For this review, take the finished solid that the model builds, in its own axes (mm). Face numbers are marked on the shaded views. A direction names the side the tool comes from. Coordinates: 2 decimals unless noted, no trailing zeros. Loops run counter-clockwise (first coordinate to the right, second up) from the corner with the lowest first, then second, coordinate; pieces in that order, holes last. Notation, with made-up numbers: (-28.5, 59) - (20.5, 59) arc R18 cw to (20.5, 84) - close; hole circle Ø7 at (46.5, 79.25). An arc over 180 degrees is marked (long way). Answer as a JSON object with one key per item and string values. Group by question number.
Item 1: Tool access review of the marked faces 5, 6 and 7: name each direction out of +Z, -Z, +X, -X, +Y, -Y from which nothing blocks a thin tool from reaching the whole face with its end or side.
Item 2: Clearance check with flat-ended pins moving along their axes: pin 1 (8 mm diameter, centred on x = 8, z = -6.5, fed in from -Y); pin 2 (1 mm diameter, centred on x = -1, z = -1, fed in from -Y); pin 3 (4 mm diameter, centred on x = -7.5, z = 3.5, fed in from -Y); pin 4 (10 mm diameter, centred on x = -3.5, y = -1.5, fed in from -Z). State where each tip first meets the part, or that it passes through.
Item 3: Mouldability with a two-part tool opening along Z and no side actions: class the marked faces 1, 2, 3 and 4 as released by +Z, released by -Z, zero draft, split by the parting line, or undercut.
Item 4: We need section C-C (z = 4.5). Give the boundary of the cut face in (x, y), then the cut area to 3 significant figures.
Item 5: To check wall thickness, follow line 1 (Y direction, x = 0, z = -3.5); line 2 (X direction, y = 3.5, z = 0.5); line 3 (Z direction, x = 6.5, y = 6). State the ranges of each line that lie inside material, in increasing order.
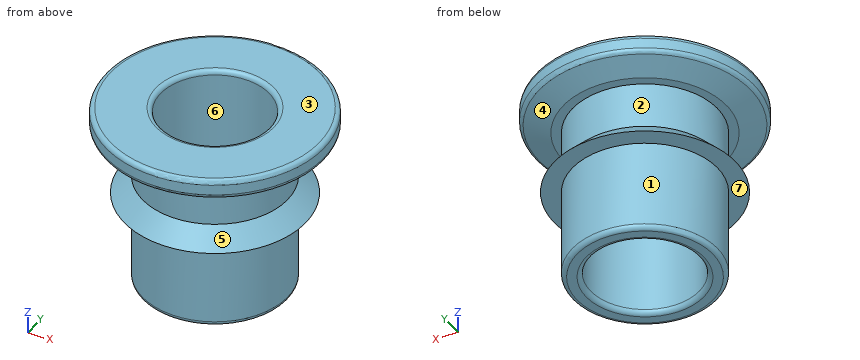
from build123d import *

# Parameters (mm, degrees)
F0_R     = 8
F0_R_2   = 6
F1_DEPTH = 10
F2_R     = 10
F2_R_2   = 6
F3_DEPTH = 2
F4_R     = 8
F4_R_2   = 6
F5_DEPTH = 5
F6_R     = 12
F6_R_2   = 6
F7_DEPTH = 3
F8_SIZE  = 1.99999
F9_SIZE2 = 3
F9_SIZE  = 1


# Not quite as in the source:
# - a fillet or chamfer that OpenCascade refuses, or shapes differently, is made with other operations: its cross-section is extruded or revolved along the edge and cut away or added
# - a fillet or chamfer is up to 0.001 mm smaller than in the source, because OpenCascade refuses the exact size


with BuildPart() as f1:
    # F0 (on Top) → F1 (new body)
    with BuildSketch(Plane.XY):
        Circle(F0_R)
        Circle(F0_R_2, mode=Mode.SUBTRACT)
    extrude(amount=-F1_DEPTH)

    # F2 (on Top) → F3 (join)
    with BuildSketch(Plane.XY):
        Circle(F2_R)
        Circle(F2_R_2, mode=Mode.SUBTRACT)
    extrude(amount=F3_DEPTH)

    # F4 (on face) → F5 (join)
    with BuildSketch(Plane.XY.offset(2)):
        Circle(F4_R)
        Circle(F4_R_2, mode=Mode.SUBTRACT)
    extrude(amount=F5_DEPTH)

    # F6 (on face) → F7 (join)
    with BuildSketch(Plane.XY.offset(7)):
        Circle(F6_R)
        Circle(F6_R_2, mode=Mode.SUBTRACT)
    extrude(amount=F7_DEPTH)

    # F8 (size 2 in the source; OpenCascade refuses exactly that, so slightly less here)
    f8_edges = [f1.edges().sort_by_distance(p)[0] for p in [
        (-10, 0, 2),
    ]]
    chamfer(f8_edges, length=F8_SIZE)

    # F9
    f9_edges = [f1.edges().sort_by_distance(p)[0] for p in [
        (-12, 0, 7),
    ]]
    f9_side = f1.faces().sort_by_distance((-12, 0, 8.5))[0]
    chamfer(f9_edges, length=F9_SIZE, length2=F9_SIZE2, reference=f9_side)

    # F10: fillet of radius 0.5 on 13 edges, made by hand

    # F10_s1 → F10_t2 (revolve, cut)
    with BuildSketch(Plane.XZ):
        with BuildLine():
            ThreePointArc((11.658113883, 7.886037961), (11.9056210926, 8.0680244677), (12, 8.36037961))
            Line((12, 8.36037961), (12, 8))
            Line((12, 8), (11.658113883, 7.886037961))
        make_face()
    revolve(axis=Axis((0, 0, 8), (0, 0, 1)), mode=Mode.SUBTRACT)

    # F10_s3 → F10_t4 (revolve, cut)
    with BuildSketch(Plane.XZ):
        with BuildLine():
            ThreePointArc((12, 9.5), (11.8535533906, 9.8535533906), (11.5, 10))
            Line((11.5, 10), (12, 10))
            Line((12, 10), (12, 9.5))
        make_face()
    revolve(axis=Axis((0, 0, 10), (0, 0, 1)), mode=Mode.SUBTRACT)

    # F10_s5 → F10_t6 (revolve, cut)
    with BuildSketch(Plane.XZ):
        with BuildLine():
            ThreePointArc((6, -9.5), (6.1464466094, -9.8535533906), (6.5, -10))
            Line((6.5, -10), (6, -10))
            Line((6, -10), (6, -9.5))
        make_face()
    revolve(axis=Axis((0, 0, -10), (0, 0, 1)), mode=Mode.SUBTRACT)

    # F10_s7 → F10_t8 (revolve, cut)
    with BuildSketch(Plane.XZ):
        with BuildLine():
            ThreePointArc((6.5, 10), (6.1464466094, 9.8535533906), (6, 9.5))
            Line((6, 9.5), (6, 10))
            Line((6, 10), (6.5, 10))
        make_face()
    revolve(axis=Axis((0, 0, 10), (0, 0, 1)), mode=Mode.SUBTRACT)

    # F10_s9 → F10_t10 (revolve, cut)
    with BuildSketch(Plane.XZ):
        with BuildLine():
            ThreePointArc((8, -9.5), (7.8535533906, -9.8535533906), (7.5, -10))
            Line((7.5, -10), (8, -10))
            Line((8, -10), (8, -9.5))
        make_face()
    revolve(axis=Axis((0, 0, -10), (0, 0, 1)), mode=Mode.SUBTRACT)


solid = f1.part
Check sheet entries:
{
 "1": {"face 5": "none", "face 6": "+Z, -Z", "face 7": "-Z"},
 "2": {"pin 1": "stops at y = -6.93", "pin 2": "stops at y = -7.98", "pin 3": "stops at y = -5.81", "pin 4": "stops at z = -10"},
 "3": {"face 1": "zero draft", "face 2": "undercut", "face 3": "released by +Z", "face 4": "undercut"},
 "4": {"outline": "circle Ø16 at (0, 0); hole circle Ø12 at (0, 0)", "area": "88.0 mm2"},
 "5": {"line 1": "y = -8 to -6, 6 to 8", "line 2": "x = -8.83 to -4.87, 4.87 to 8.83", "line 3": "z = 0 to 1.15, 7 to 10"}
}
